```python
from build123d import *

# Parameters (mm, degrees)
SKIZZE1_W                       = 36
SKIZZE1_H                       = 70
AUFSATZ_LINEAR_AUSTRAGEN1_DEPTH = 10
SKIZZE2_R                       = 1.5
SCHNITT_LINEAR_AUSTRAGEN1_DEPTH = 71
SKIZZE3_R                       = 2
SCHNITT_LINEAR_AUSTRAGEN2_DEPTH = 6
SKIZZE4_R                       = 2
SCHNITT_LINEAR_AUSTRAGEN3_DEPTH = 6


with BuildPart() as part:
    # Skizze1 → Aufsatz-Linear austragen1 (new body)
    with BuildSketch(Plane.XY):
        with Locations((4.904225341, 35)):
            Rectangle(SKIZZE1_W, SKIZZE1_H)
        with BuildLine():
            Line((17.904225341, 51.106779598), (17.904225341, 18.893220402))
            ThreePointArc((17.904225341, 18.893220402), (17.153006461, 17.92466067), (16.028009433, 18.411301652))
            Line((16.028009433, 18.411301652), (7.169280654, 34.51808125))
            ThreePointArc((7.169280654, 34.51808125), (7.045496562, 35), (7.169280654, 35.48191875))
            Line((7.169280654, 35.48191875), (16.028009433, 51.588698348))
            ThreePointArc((16.028009433, 51.588698348), (17.153006461, 52.07533933), (17.904225341, 51.106779598))
        make_face(mode=Mode.SUBTRACT)
        with BuildLine():
            Line((-8.095774659, 51.106779598), (-8.095774659, 18.893220402))
            ThreePointArc((-8.095774659, 18.893220402), (-7.344555779, 17.92466067), (-6.21955875, 18.411301652))
            Line((-6.21955875, 18.411301652), (2.639170029, 34.51808125))
            ThreePointArc((2.639170029, 34.51808125), (2.76295412, 35), (2.639170029, 35.48191875))
            Line((2.639170029, 35.48191875), (-6.21955875, 51.588698348))
            ThreePointArc((-6.21955875, 51.588698348), (-7.344555779, 52.07533933), (-8.095774659, 51.106779598))
        make_face(mode=Mode.SUBTRACT)
        with BuildLine():
            Line((-6.053662963, 60), (16.441312792, 60))
            ThreePointArc((16.441312792, 60), (17.312422464, 59.491088524), (17.296896718, 58.482335877))
            Line((17.296896718, 58.482335877), (5.780402017, 39.448125623))
            ThreePointArc((5.780402017, 39.448125623), (4.914343105, 38.96584461), (4.058577468, 39.466162699))
            Line((4.058577468, 39.466162699), (-6.919903585, 58.500372954))
            ThreePointArc((-6.919903585, 58.500372954), (-6.919580698, 59.500186442), (-6.053662963, 60))
        make_face(mode=Mode.SUBTRACT)
        with BuildLine():
            Line((-6.25411364, 10), (16.240977478, 10))
            ThreePointArc((16.240977478, 10), (17.110316116, 10.505783111), (17.100261151, 11.511499334))
            Line((17.100261151, 11.511499334), (5.769851759, 30.545807203))
            ThreePointArc((5.769851759, 30.545807203), (4.907341379, 31.034302663), (4.048001406, 30.540251269))
            Line((4.048001406, 30.540251269), (-7.116680319, 11.5059434))
            ThreePointArc((-7.116680319, 11.5059434), (-7.121853059, 10.502980584), (-6.25411364, 10))
        make_face(mode=Mode.SUBTRACT)
    extrude(amount=AUFSATZ_LINEAR_AUSTRAGEN1_DEPTH)

    # Skizze2 → Schnitt-Linear austragen1 (cut, through all)
    with BuildSketch(Plane(origin=(0, 70, 0), x_dir=(1, 0, 0), z_dir=(0, 1, 0))):
        with Locations((5, -5)):
            Circle(SKIZZE2_R)
    extrude(amount=-SCHNITT_LINEAR_AUSTRAGEN1_DEPTH, mode=Mode.SUBTRACT)

    # Skizze3 → Schnitt-Linear austragen2 (cut)
    with BuildSketch(Plane(origin=(0, 70, 0), x_dir=(1, 0, 0), z_dir=(0, 1, 0))):
        with Locations((5, -5)):
            Circle(SKIZZE3_R)
    extrude(amount=-SCHNITT_LINEAR_AUSTRAGEN2_DEPTH, mode=Mode.SUBTRACT)

    # Skizze4 → Schnitt-Linear austragen3 (cut)
    with BuildSketch(Plane.XZ):
        with Locations((5, 5)):
            Circle(SKIZZE4_R)
    extrude(amount=-SCHNITT_LINEAR_AUSTRAGEN3_DEPTH, mode=Mode.SUBTRACT)


solid = part.part
```
For this review, take the finished solid that the model builds, in its own axes (mm). A direction names the side the tool comes from. Give positions to 0.01 mm unless a question says otherwise; leave off trailing zeros. Write each loop counter-clockwise with the first axis right and the second up, starting at its lowest first coordinate (ties: lowest second). Pieces come first, ordered by that corner, then holes. Notation, with made-up numbers: M 19.5,-22 L 41.5,-22 A18 cw 41.5,-13 Z; hole C 19,83 d10. An arc over 180 degrees is marked long. Answer as CSV lines item,"result".
1. Consider section B-B, the plane x = 5. Count the separate pieces of the cut face and the enclosed holes in it, then the cut area to 3 significant figures.
Findings:
separate pieces,"6"
enclosed holes,"0"
area,"184 mm2"
2. Consider section C-C, the plane y = 47. Write out the cut boundary in (x, z).
Findings:
outline,"M -13.1,0 L -8.1,0 L -8.1,10 L -13.1,10 Z; M -3.7,0 L -0.29,0 L -0.29,10 L -3.7,10 Z; M 10.35,0 L 13.5,0 L 13.5,10 L 10.35,10 Z; M 17.9,0 L 22.9,0 L 22.9,10 L 17.9,10 Z"
3. For faces 1 (the cylindrical face through (4.922, 31.034, 8.053)), 2 (the flat face through (4.7, 70, 2.7)), list the 3-axis set-ups (+Z, -Z, +X, -X, +Y, -Y) from which the entire face can be reached by the end or side of a thin tool; tool diameter is ignored.
Findings:
face 1,"+Z, -Z"
face 2,"+Z, -Z, +X, -X, +Y"
4. Consider section D-D, the plane x = 0.5. Write out the cut boundary in (y, z), then the cut area to 3 significant figures.
Findings:
outline,"M 0,0 L 10,0 L 10,10 L 0,10 Z; M 24.49,0 L 30.63,0 L 30.63,10 L 24.49,10 Z; M 39.37,0 L 45.64,0 L 45.64,10 L 39.37,10 Z; M 60,0 L 70,0 L 70,10 L 60,10 Z"
area,"324 mm2"
5. Draft analysis for pull direction X (two halves, no side actions). For faces 3 (the cylindrical face through (3, 3, 5)), 4 (the cylindrical face through (17.1, 10.49, 4.93)), 5 (the flat face through (5, 35, 10)), 6 (the flat face through (22.904, 35, 5)), state which applies: +X half, -X half, draft (parallel to the pull), parting line (faces both ways), or undercut.
Findings:
face 3,"undercut"
face 4,"undercut"
face 5,"draft"
face 6,"+X half"
6. Consider section A-A, the plane z = 1. Write out the cut boundary in (x, y).
Findings:
outline,"M -13.1,0 L 22.9,0 L 22.9,70 L -13.1,70 Z; hole M -8.1,18.89 A1 ccw -6.22,18.41 L 2.64,34.52 A1 ccw 2.64,35.48 L -6.22,51.59 A1 ccw -8.1,51.11 Z; hole M -7.12,11.51 A1 ccw -6.25,10 L 16.24,10 A1 ccw 17.1,11.51 L 5.77,30.55 A1 ccw 4.05,30.54 Z; hole M -6.92,58.5 L 4.06,39.47 A1 ccw 5.78,39.45 L 17.3,58.48 A1 ccw 16.44,60 L -6.05,60 A1 ccw Z; hole M 7.17,34.52 L 16.03,18.41 A1 ccw 17.9,18.89 L 17.9,51.11 A1 ccw 16.03,51.59 L 7.17,35.48 A1 ccw Z"
7. Wall thickness on line 1 (Z direction, x = 5, y = 7.8); line 2 (Y direction, x = -2.5, z = 7.75); line 3 (X direction, y = 52, z = 9): over which ranges is each line inside the solid? List them lowest first.
Findings:
line 1,"z = 0 to 3.5, 6.5 to 10"
line 2,"y = 0 to 10, 19.38 to 25.17, 44.83 to 50.84, 60 to 70"
line 3,"x = -13.1 to -7.55, -6.65 to -3.17, 13.37 to 16.45, 17.35 to 22.9"
8. For pin 1 (3 mm diameter, centred on x = 2.5, z = 7.5, fed in from -Y), flat-tipped, find the tip position at first contact; note if it passes through.
Findings:
pin 1,"stops at y = 0"
